```python
from build123d import *

# Parameters (mm, degrees)
F0_W      = 56.4
F0_H      = 56.4
F1_DEPTH  = 54.1
F2_R      = 19.05
F3_DEPTH  = 1.6
F4_R      = 3.175
F5_DEPTH  = 20
F6_R      = 2.6
F7_DEPTH  = 54.101
F9_DEPTH  = 15
F10_R     = 4.6
F11_W     = 12
F11_H     = 12
F12_DEPTH = 49.1
F13_R     = 5
F14_SIZE  = 1


with BuildPart() as f1:
    # F0 (on Front) → F1 (new body)
    with BuildSketch(Plane.XZ):
        Rectangle(F0_W, F0_H)
    extrude(amount=-F1_DEPTH)

    # F2 (on face) → F3 (join)
    with BuildSketch(Plane.XZ):
        Circle(F2_R)
    extrude(amount=F3_DEPTH)

    # F4 (on face) → F5 (join)
    with BuildSketch(Plane.XZ):
        Circle(F4_R)
    extrude(amount=F5_DEPTH)

    # F6 (on face) → F7 (cut, through all)
    with BuildSketch(Plane.XZ):
        with Locations((23.57, 23.57)):
            Circle(F6_R)
        with Locations((-23.57, 23.57)):
            Circle(F6_R)
        with Locations((23.57, -23.57)):
            Circle(F6_R)
        with Locations((-23.57, -23.57)):
            Circle(F6_R)
    extrude(amount=-F7_DEPTH, mode=Mode.SUBTRACT)

    # F8 (on face) → F9 (cut)
    with BuildSketch(Plane.XZ.offset(20)):
        with BuildLine():
            Line((-2.625, -1.7860571099), (-2.625, 1.7860571099))
            ThreePointArc((-2.625, 1.7860571099), (-3.175, 0), (-2.625, -1.7860571099))
        make_face()
    extrude(amount=-F9_DEPTH, mode=Mode.SUBTRACT)

    # F10
    f10_edges = [f1.edges().sort_by_distance(p)[0] for p in [
        (-28.2, 27.05, 28.2),
        (-28.2, 27.05, -28.2),
        (28.2, 27.05, 28.2),
        (28.2, 27.05, -28.2),
    ]]
    fillet(f10_edges, radius=F10_R)

    # F11 (on face) → F12 (cut)
    with BuildSketch(Plane(origin=(0, 54.1, 0), x_dir=(-1, 0, 0), z_dir=(0, 1, 0))):
        with Locations((22.2, 22.2)):
            Rectangle(F11_W, F11_H)
        with Locations((-22.2, 22.2)):
            Rectangle(F11_W, F11_H)
        with Locations((22.2, -22.2)):
            Rectangle(F11_W, F11_H)
        with Locations((-22.2, -22.2)):
            Rectangle(F11_W, F11_H)
    extrude(amount=-F12_DEPTH, mode=Mode.SUBTRACT)

    # F13
    f13_edges = [f1.edges().sort_by_distance(p)[0] for p in [
        (-16.2, 29.55, 28.2),
        (-16.2, 29.55, 16.2),
        (-28.2, 29.55, 16.2),
        (16.2, 29.55, 28.2),
        (16.2, 29.55, 16.2),
        (28.2, 29.55, 16.2),
        (28.2, 29.55, -16.2),
        (16.2, 29.55, -16.2),
        (16.2, 29.55, -28.2),
        (-16.2, 29.55, -28.2),
        (-16.2, 29.55, -16.2),
        (-28.2, 29.55, -16.2),
    ]]
    fillet(f13_edges, radius=F13_R)

    # F14
    f14_edges = [f1.edges().sort_by_distance(p)[0] for p in [
        (0, 54.1, 28.2),
    ]]
    chamfer(f14_edges, length=F14_SIZE)


solid = f1.part
```
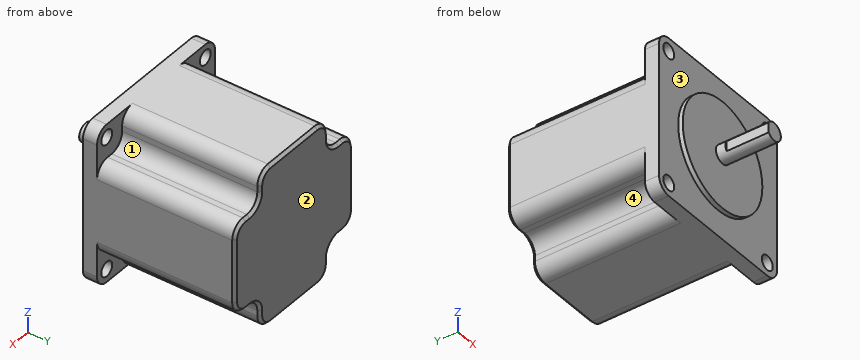
The model under review builds one solid part; all positions refer to its coordinate system, in mm. Face numbers are marked on the shaded views. A direction names the side the tool comes from. Give positions to 0.01 mm unless a question says otherwise; leave off trailing zeros. Write each loop counter-clockwise with the first axis right and the second up, starting at its lowest first coordinate (ties: lowest second). Pieces come first, ordered by that corner, then holes.
(1) For P1, Ø3, axis at x = -23.57, z = 23.57, coming from the -Y side; P2, Ø2, axis at y = 19, z = 22, coming from the -X side; P3, Ø2, axis at y = 18.5, z = -22, coming from the +X side; P4, Ø1, axis at x = -22, y = 25.5, coming from the +Z side, all flat-tipped, find the tip position at first contact; note any pin that passes through.
(2) Consider section C-C, the plane x = 0. Give the boundary of the cut face in (y, z) (3 decimals), and give its area (3 significant figures).
(3) Consider section B-B, the plane z = 0. Give the boundary of the cut face in (x, y) (3 decimals).
(4) To check wall thickness, follow L1, parallel to Z at x = -23.57, y = 1.3; L2, parallel to Y at x = -7.5, z = -6; L3, parallel to Y at x = 20, z = -20. State the ranges of each line that lie inside material, in increasing order.
(5) Consider section A-A, the plane y = 13.5. Give the boundary of the cut face in (x, z).
(6) Tool access review of the marked faces 1, 2, 3 and 4: name each direction out of +Z, -Z, +X, -X, +Y, -Y from which nothing blocks a thin tool from reaching the whole face with its end or side.
(7) Consider section D-D, the plane z = -9.5. Give the boundary of the cut face in (x, y), and give its area (3 significant figures).
Returned:
1. P1: passes through
1. P2: stops at x = -16.2
1. P3: stops at x = 16.2
1. P4: stops at z = 16.2
2. outline: (-20, -3.175) - (-1.6, -3.175) - (-1.6, -19.05) - (0, -19.05) - (0, -28.2) - (53.1, -28.2) - (54.1, -27.2) - (54.1, 27.2) - (53.1, 28.2) - (0, 28.2) - (0, 19.05) - (-1.6, 19.05) - (-1.6, 3.175) - (-20, 3.175) - close
2. area: 3,230 mm2
3. outline: (-28.2, 0) - (-19.05, 0) - (-19.05, -1.6) - (-3.175, -1.6) - (-3.175, -5) - (-2.625, -5) - (-2.625, -20) - (3.175, -20) - (3.175, -1.6) - (19.05, -1.6) - (19.05, 0) - (28.2, 0) - (28.2, 53.1) - (27.2, 54.1) - (-27.2, 54.1) - (-28.2, 53.1) - close
4. L1: z = -28.2 to -26.17, -20.97 to 20.97, 26.17 to 28.2
4. L2: y = -1.6 to 54.1
4. L3: y = 0 to 5
5. outline: (-28.2, -11.2) arc R5 ccw to (-23.2, -16.2) - (-21.2, -16.2) arc R5 cw to (-16.2, -21.2) - (-16.2, -23.2) arc R5 ccw to (-11.2, -28.2) - (11.2, -28.2) arc R5 ccw to (16.2, -23.2) - (16.2, -21.2) arc R5 cw to (21.2, -16.2) - (23.2, -16.2) arc R5 ccw to (28.2, -11.2) - (28.2, 11.2) arc R5 ccw to (23.2, 16.2) - (21.2, 16.2) arc R5 cw to (16.2, 21.2) - (16.2, 23.2) arc R5 ccw to (11.2, 28.2) - (-11.2, 28.2) arc R5 ccw to (-16.2, 23.2) - (-16.2, 21.2) arc R5 cw to (-21.2, 16.2) - (-23.2, 16.2) arc R5 ccw to (-28.2, 11.2) - close
6. face 1: +Z, +X, +Y
6. face 2: +Z, -Z, +X, -X, +Y
6. face 3: -Y
6. face 4: -Z, -X, +Y
7. outline: (-28.2, 0) - (-16.51, 0) - (-16.51, -1.6) - (16.51, -1.6) - (16.51, 0) - (28.2, 0) - (28.2, 53.1) - (27.2, 54.1) - (-27.2, 54.1) - (-28.2, 53.1) - close
7. area: 3,100 mm2
